Geometry: see drawing. Coordinates: mm, zero at the bounding-box minimum. Round coordinates to 2 decimals unless told otherwise and drop trailing zeros. Write each loop counter-clockwise with the first axis right and the second up, starting at its lowest first coordinate (ties: lowest second). Pieces come first, ordered by that corner, then holes. Notation, with made-up numbers: (75, 39) - (130, 39) arc R20 ccw to (130, 51) - close; hole circle Ø1 at (46, 19). An arc over 180 degrees is marked (long way). Use a Markdown table: item, result. Add a question column.
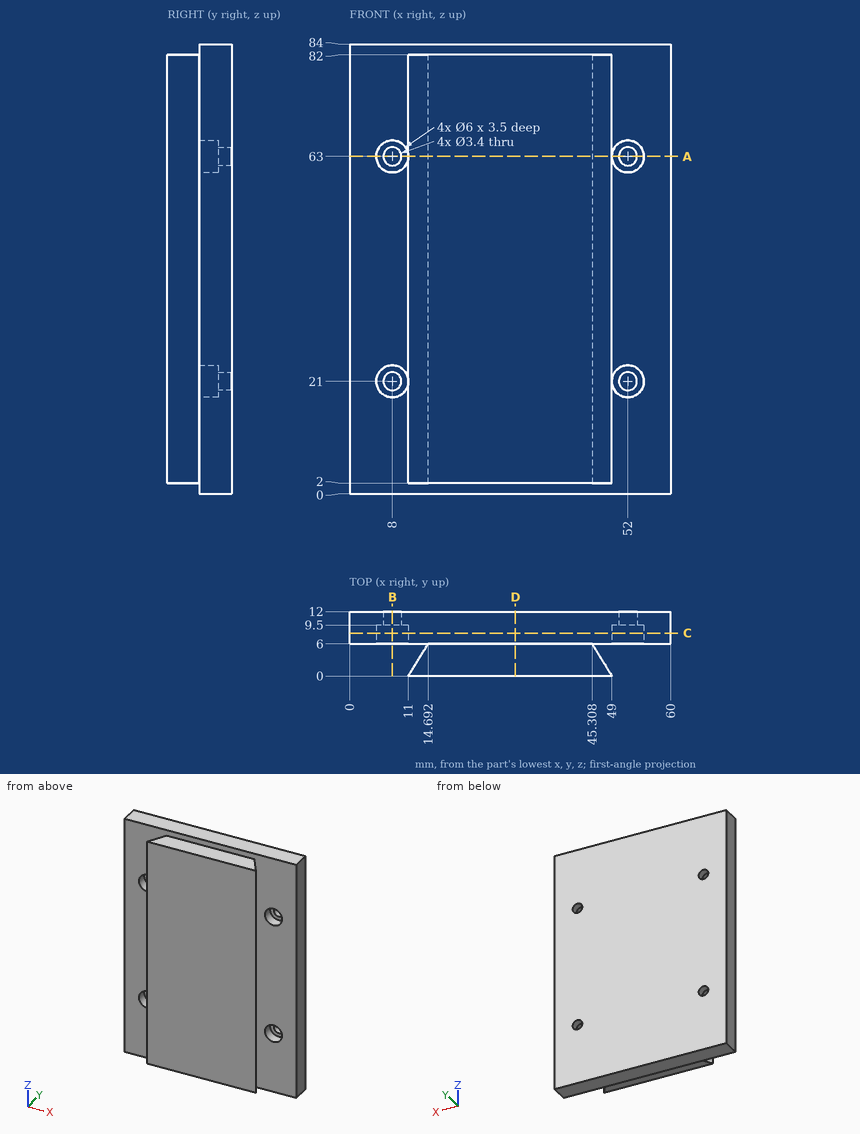
1) Section A-A, the plane z = 63. Return the cut outline in (x, y), then the cut area to 3 significant figures.
2) Section D-D, the plane x = 31. Return the cut outline in (y, z).
3) Pin query (flat end, axial travel): P1, Ø1, axis at y = 7.5, z = 64, coming from the -X side; P2, Ø1.8, axis at x = 8, z = 20, coming from the -Y side; P3, Ø1, axis at x = 14, y = 2, coming from the +Z side; P4, Ø1.8, axis at x = 37, y = 4, coming from the -Z side. Return the tip coordinate at first contact, or that it passes through.
4) Material intervals for L1, parallel to Z at x = 52, y = 11.15; L2, parallel to Z at x = 52, y = 6.9; L3, parallel to X at y = 7.4, z = 63, sorted ascending. Write a range as from..to.
5) Section B-B, the plane x = 8. Return the cut outline in (y, z).
6) Section C-C, the plane y = 8. Return the cut outline in (x, z), then the cut area to 3 significant figures.
Output values:
| question | item | result |
|---|---|---|
| 1 | outline | (0, 6) - (5, 6) - (5, 9.5) - (6.3, 9.5) - (6.3, 12) - (0, 12) - close; (9.7, 9.5) - (11, 9.5) - (11, 6) - (14.69, 6) - (11, 0) - (49, 0) - (45.31, 6) - (49, 6) - (49, 9.5) - (50.3, 9.5) - (50.3, 12) - (9.7, 12) - close; (53.7, 9.5) - (55, 9.5) - (55, 6) - (60, 6) - (60, 12) - (53.7, 12) - close |
| 1 | area | 507 mm^2 |
| 2 | outline | (0, 2) - (6, 2) - (6, 0) - (12, 0) - (12, 84) - (6, 84) - (6, 82) - (0, 82) - close |
| 3 | P1 | stops at x = 0 |
| 3 | P2 | stops at y = 9.5 |
| 3 | P3 | stops at z = 82 |
| 3 | P4 | stops at z = 2 |
| 4 | L1 | z = 0..19.3, 22.7..61.3, 64.7..84 |
| 4 | L2 | z = 0..18, 24..60, 66..84 |
| 4 | L3 | x = 0..5, 11..49, 55..60 |
| 5 | outline | (6, 0) - (12, 0) - (12, 19.3) - (9.5, 19.3) - (9.5, 18) - (6, 18) - close; (6, 24) - (9.5, 24) - (9.5, 22.7) - (12, 22.7) - (12, 61.3) - (9.5, 61.3) - (9.5, 60) - (6, 60) - close; (6, 66) - (9.5, 66) - (9.5, 64.7) - (12, 64.7) - (12, 84) - (6, 84) - close |
| 6 | outline | (0, 0) - (60, 0) - (60, 84) - (0, 84) - close; hole circle Ø6 at (8, 21); hole circle Ø6 at (8, 63); hole circle Ø6 at (52, 21); hole circle Ø6 at (52, 63) |
| 6 | area | 4,930 mm^2 |
